Read the model definition and answer for the solid it produces. Units are mm, in the model's axes. A direction names the side the tool comes from. Round coordinates to 2 decimals unless told otherwise and drop trailing zeros. Write each loop counter-clockwise with the first axis right and the second up, starting at its lowest first coordinate (ties: lowest second). Pieces come first, ordered by that corner, then holes. Notation, with made-up numbers: M 52,-20.75 L 69,-20.75 A21 cw 69,-2.75 Z; hole C 60,65 d8. An arc over 180 degrees is marked long. Use one line per item in the form item = value. Start each with the question number.
```python
from build123d import *

# Parameters (mm, degrees)
F0_W      = 372
F0_H      = 272
F1_DEPTH  = 15
F2_W      = 372
F2_H      = 272
F3_DEPTH  = 2
F5_DEPTH  = 31
F7_DEPTH  = 2
F9_DEPTH  = 23
F11_DEPTH = 2
F12_W     = 370
F12_H     = 270
F13_DEPTH = 73
F15_DEPTH = 13
F17_DEPTH = 13
F18_R     = 2


with BuildPart() as f1:
    # F0 (on Top) → F1 (new body)
    with BuildSketch(Plane.XY):
        Rectangle(F0_W, F0_H)
    extrude(amount=F1_DEPTH)

    # F2 (on face) → F3 (join)
    with BuildSketch(Plane.XY.offset(15)):
        with BuildLine():
            Line((-190, -150), (190, -150))
            ThreePointArc((190, -150), (197.0710678119, -147.0710678119), (200, -140))
            Line((200, -140), (200, 140))
            ThreePointArc((200, 140), (197.0710678119, 147.0710678119), (190, 150))
            Line((190, 150), (-190, 150))
            ThreePointArc((-190, 150), (-197.0710678119, 147.0710678119), (-200, 140))
            Line((-200, 140), (-200, -140))
            ThreePointArc((-200, -140), (-197.0710678119, -147.0710678119), (-190, -150))
        make_face()
        Rectangle(F2_W, F2_H, mode=Mode.SUBTRACT)
        Rectangle(F2_W, F2_H)
    extrude(amount=F3_DEPTH)

    # F4 (on face) → F5 (join)
    with BuildSketch(Plane.XY.offset(17)):
        Polygon((157, -137), (187, -137), (187, -107), (200, -107), (200, -105), (187, -105), (187, 105), (200, 105), (200, 107), (187, 107), (187, 137), (157, 137), (157, 150), (155, 150), (155, 137), (-155, 137), (-155, 150), (-157, 150), (-157, 137), (-187, 137), (-187, 107), (-200, 107), (-200, 105), (-187, 105), (-187, -105), (-200, -105), (-200, -107), (-187, -107), (-187, -137), (-157, -137), (-157, -150), (-155, -150), (-155, -137), (155, -137), (155, -150), (157, -150), align=None)
    extrude(amount=F5_DEPTH)

    # F6 (on face) → F7 (join)
    with BuildSketch(Plane.XY.offset(48)):
        with BuildLine():
            Line((190, 150), (-190, 150))
            ThreePointArc((-190, 150), (-197.0710678119, 147.0710678119), (-200, 140))
            Line((-200, 140), (-200, -140))
            ThreePointArc((-200, -140), (-197.0710678119, -147.0710678119), (-190, -150))
            Line((-190, -150), (190, -150))
            ThreePointArc((190, -150), (197.0710678119, -147.0710678119), (200, -140))
            Line((200, -140), (200, 140))
            ThreePointArc((200, 140), (197.0710678119, 147.0710678119), (190, 150))
        make_face()
    extrude(amount=F7_DEPTH)

    # F8 (on face) → F9 (join)
    with BuildSketch(Plane.XY.offset(50)):
        with BuildLine():
            Line((-185.3079227659, -137), (185.3079227659, -137))
            Line((185.3079227659, -137), (197.8531877713, -146.1909160735))
            ThreePointArc((197.8531877713, -146.1909160735), (198.4340605379, -145.3727667773), (198.9300207482, -144.5005254622))
            Line((198.9300207482, -144.5005254622), (187, -135.7603498338))
            Line((187, -135.7603498338), (187, 135.7603498338))
            Line((187, 135.7603498338), (198.9300207482, 144.5005254622))
            ThreePointArc((198.9300207482, 144.5005254622), (198.4340605379, 145.3727667773), (197.8531877713, 146.1909160735))
            Line((197.8531877713, 146.1909160735), (185.3079227659, 137))
            Line((185.3079227659, 137), (-185.3079227659, 137))
            Line((-185.3079227659, 137), (-197.8531877713, 146.1909160735))
            ThreePointArc((-197.8531877713, 146.1909160735), (-198.4340605379, 145.3727667773), (-198.9300207482, 144.5005254622))
            Line((-198.9300207482, 144.5005254622), (-187, 135.7603498338))
            Line((-187, 135.7603498338), (-187, -135.7603498338))
            Line((-187, -135.7603498338), (-198.9300207482, -144.5005254622))
            ThreePointArc((-198.9300207482, -144.5005254622), (-198.4340605379, -145.3727667773), (-197.8531877713, -146.1909160735))
            Line((-197.8531877713, -146.1909160735), (-185.3079227659, -137))
        make_face()
    extrude(amount=F9_DEPTH)

    # F10 (on face) → F11 (join)
    with BuildSketch(Plane.XY.offset(73)):
        with BuildLine():
            Line((-190, -150), (190, -150))
            ThreePointArc((190, -150), (197.0710678119, -147.0710678119), (200, -140))
            Line((200, -140), (200, 140))
            ThreePointArc((200, 140), (197.0710678119, 147.0710678119), (190, 150))
            Line((190, 150), (-190, 150))
            ThreePointArc((-190, 150), (-197.0710678119, 147.0710678119), (-200, 140))
            Line((-200, 140), (-200, -140))
            ThreePointArc((-200, -140), (-197.0710678119, -147.0710678119), (-190, -150))
        make_face()
    extrude(amount=F11_DEPTH)

    # F12 (on face) → F13 (cut)
    with BuildSketch(Plane.XY.offset(75)):
        Rectangle(F12_W, F12_H)
    extrude(amount=-F13_DEPTH, mode=Mode.SUBTRACT)

    # F14 (on face) → F15 (join, through all)
    with BuildSketch(Plane(origin=(-187, 0, 0), x_dir=(0, -1, 0), z_dir=(-1, 0, 0))):
        with BuildLine():
            Line((-63, 18), (63, 18))
            ThreePointArc((63, 18), (65.8284271247, 19.1715728753), (67, 22))
            Line((67, 22), (67, 48))
            Line((67, 48), (65, 48))
            Line((65, 48), (65, 22))
            ThreePointArc((65, 22), (64.4142135624, 20.5857864376), (63, 20))
            Line((63, 20), (-63, 20))
            ThreePointArc((-63, 20), (-64.4142135624, 20.5857864376), (-65, 22))
            Line((-65, 22), (-65, 48))
            Line((-65, 48), (-67, 48))
            Line((-67, 48), (-67, 22))
            ThreePointArc((-67, 22), (-65.8284271247, 19.1715728753), (-63, 18))
        make_face()
    extrude(amount=F15_DEPTH)

    # F16 (on face) → F17 (join, through all)
    with BuildSketch(Plane.YZ.offset(187)):
        with BuildLine():
            ThreePointArc((63, 18), (65.8284271247, 19.1715728753), (67, 22))
            Line((67, 22), (67, 48))
            Line((67, 48), (65, 48))
            Line((65, 48), (65, 22))
            ThreePointArc((65, 22), (64.4142135624, 20.5857864376), (63, 20))
            Line((63, 20), (-63, 20))
            ThreePointArc((-63, 20), (-64.4142135624, 20.5857864376), (-65, 22))
            Line((-65, 22), (-65, 48))
            Line((-65, 48), (-67, 48))
            Line((-67, 48), (-67, 22))
            ThreePointArc((-67, 22), (-65.8284271247, 19.1715728753), (-63, 18))
            Line((-63, 18), (63, 18))
        make_face()
    extrude(amount=F17_DEPTH)

    # F18
    f18_edges = [f1.edges().sort_by_distance(p)[0] for p in [
        (-185, -135, 38.5),
        (185, -135, 38.5),
        (185, 135, 38.5),
        (0, 135, 2),
        (185, 0, 2),
        (0, -135, 2),
        (-185, 0, 2),
        (-185, 135, 38.5),
        (187, -137, 32.5),
        (187, 137, 32.5),
        (-187, 137, 32.5),
        (-187, -137, 32.5),
        (186, 0, 0),
        (0, 136, 0),
        (186, 136, 7.5),
        (0, -136, 0),
        (186, -136, 7.5),
        (-186, -136, 7.5),
        (-186, 0, 0),
        (-186, 136, 7.5),
    ]]
    fillet(f18_edges, radius=F18_R)


solid = f1.part
```
Q1. For a pull along Y with two mould halves and no side action, classify faces 4 (the face through (157, 143, 32)), 5 (the face through (171, 137, 32)), 6 (the face through (-193, 65, 35)) as +Y half, -Y half, draft (parallel to the pull), parting line (faces both ways), or undercut.
Q2. A tool of negligible diameter and unlimited length cuts with its end or side. For faces 1 (the face through (-186, -2, 8)), 2 (the face through (193, -86, 48)), 3 (the face through (-194, -86, 48)), from which of +Z, -Z, +X, -X, +Y, -Y can it reach the whole face along a straight path? Write none if from no direction.
Q3. Find section B-B on z = 57. Write down the section's boundary in (x, y).
Q4. Each of these flat-tipped pins is pushed along its axis until it touches: pin 1 Ø6.5 at (x, y) = (-190.5, -84.5) entering from -Z; pin 2 Ø14.5 at (y, z) = (-143.5, 26.5) entering from +X; pin 3 Ø6 at (x, z) = (29.5, 20.5) entering from +Y. Where does it stop, or does it pass through?
Q5. Straight lines are drawn through the part: line 1 (Y direction, x = 21.5, z = 26.5); line 2 (X direction, y = 103, z = 67); line 3 (X direction, y = 119.5, z = 49). For each, find the intervals that lie inside material, in ascending order. Write a range as [from, to].
Response:
q1.face_4 = draft
q1.face_5 = +Y half
q1.face_6 = undercut
q2.face_1 = -Z, -X, +Y, -Y
q2.face_2 = +X
q2.face_3 = -X
q3.outline = M -198.93,-144.5 A10 ccw -197.85,-146.19 L -185.31,-137 L 185.31,-137 L 197.85,-146.19 A10 ccw 198.93,-144.5 L 187,-135.76 L 187,135.76 L 198.93,144.5 A10 ccw 197.85,146.19 L 185.31,137 L -185.31,137 L -197.85,146.19 A10 ccw -198.93,144.5 L -187,135.76 L -187,-135.76 Z; hole M -185,-133 A2 ccw -183,-135 L 183,-135 A2 ccw 185,-133 L 185,133 A2 ccw 183,135 L -183,135 A2 ccw -185,133 Z
q4.pin_1 = 15
q4.pin_2 = 186.56
q4.pin_3 = 137
q5.line_1 = [-137, -135], [135, 137]
q5.line_2 = [-187, -185], [185, 187]
q5.line_3 = [-200, -185], [185, 200]
